from build123d import *

# Parameters (mm, degrees)
SKETCH1_W           = 90
SKETCH1_H           = 60
SKETCH1_R           = 2.3
BOSS_EXTRUDE1_DEPTH = 15
SKETCH2_R           = 9
CUT_EXTRUDE1_DEPTH  = 72


with BuildPart() as part:
    # Sketch1 → Boss-Extrude1 (new body)
    with BuildSketch(Plane.XY):
        Rectangle(SKETCH1_W, SKETCH1_H)
        with Locations((-35, -20)):
            Circle(SKETCH1_R, mode=Mode.SUBTRACT)
        with Locations(Location((35, -20, 0), (0, 0, 180))):
            Circle(SKETCH1_R, mode=Mode.SUBTRACT)
        with Locations((35, 20)):
            Circle(SKETCH1_R, mode=Mode.SUBTRACT)
        with Locations(Location((-35, 20, 0), (0, 0, 180))):
            Circle(SKETCH1_R, mode=Mode.SUBTRACT)
    extrude(amount=BOSS_EXTRUDE1_DEPTH)

    # Sketch2 → Cut-Extrude1 (cut)
    with BuildSketch(Plane.XZ.offset(30)):
        with Locations((0, 15)):
            Circle(SKETCH2_R)
    extrude(amount=-CUT_EXTRUDE1_DEPTH, mode=Mode.SUBTRACT)


solid = part.part
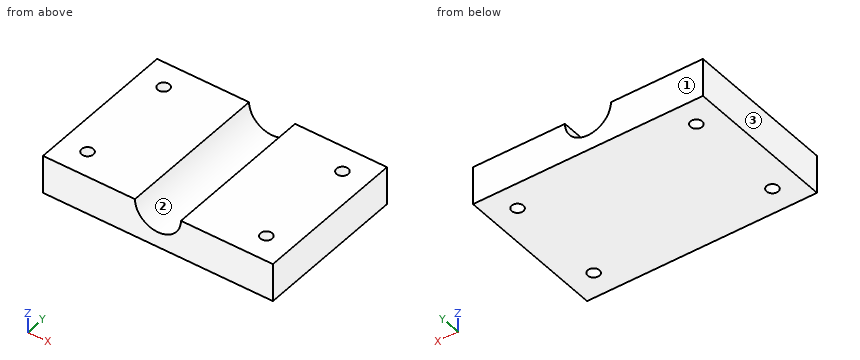
Can you work these out from the model? Positions are in its coordinate system, mm. Face numbers are marked on the shaded views. Round coordinates to 2 decimals unless told otherwise and drop trailing zeros. Loops run counter-clockwise (first coordinate to the right, second up) from the corner with the lowest first, then second, coordinate; pieces in that order, holes last. Notation, with made-up numbers: (-7, -28) - (35, -28) arc R33 ccw to (35, 9) - close; hole circle Ø4 at (59, 62.5). An arc over 180 degrees is marked (long way). Answer in a Markdown table with one row per item. Add a question column.
Q1. I want a section at B-B on y = -15.5. List the corners of the cut face in (x, z) for me, and give its area (3 significant figures).
Q2. For pin 1 Ø1.5 at (x, y) = (-28.5, -6) entering from -Z, with a flat end and sliding along its axis, tell me the tip position at first contact or that it passes through.
Q3. I need wall thicknesses on L1, parallel to Y at x = 35, z = 10; L2, parallel to Y at x = -34, z = 9.5; L3, parallel to X at y = -12.5, z = 12. Which ranges of each line are inside material? Lowest first, please.
Q4. I want a section at A-A on z = 12.75. List the corners of the cut face in (x, y) for me.
Q5. I want a section at C-C on x = 0. List the corners of the cut face in (y, z) for me.
Q6. We'd pull the mould along X, two halves only. Please class the marked faces 1, 2 and 3: pulls with the +X half, pulls with the -X half, needs draft (parallel to the pull), parting line crosses it, or undercut.
A:
| question | item | result |
|---|---|---|
| 1 | outline | (-45, 0) - (45, 0) - (45, 15) - (9, 15) arc R9 cw to (-9, 15) - (-45, 15) - close |
| 1 | area | 1,220 mm^2 |
| 2 | pin 1 | z = 0 |
| 3 | L1 | -30 to -22.3, -17.7 to 17.7, 22.3 to 30 |
| 3 | L2 | -30 to -22.07, -17.93 to 17.93, 22.07 to 30 |
| 3 | L3 | -45 to -8.49, 8.49 to 45 |
| 4 | outline | (-45, -30) - (-8.71, -30) - (-8.71, 30) - (-45, 30) - close; (8.71, -30) - (45, -30) - (45, 30) - (8.71, 30) - close; hole circle Ø4.6 at (-35, -20); hole circle Ø4.6 at (-35, 20); hole circle Ø4.6 at (35, -20); hole circle Ø4.6 at (35, 20) |
| 5 | outline | (-30, 0) - (30, 0) - (30, 6) - (-30, 6) - close |
| 6 | face 1 | needs draft |
| 6 | face 2 | undercut |
| 6 | face 3 | pulls with the -X half |
